Check sheet for the modelled part. Datum: model origin and axes. Units: mm. A direction names the side the tool comes from. Round coordinates to 2 decimals unless told otherwise and drop trailing zeros. Loops run counter-clockwise (first coordinate to the right, second up) from the corner with the lowest first, then second, coordinate; pieces in that order, holes last. Notation, with made-up numbers: (41, -25) - (93, -25) arc R30 ccw to (93, 13) - close; hole circle Ø11 at (75.5, 61). An arc over 180 degrees is marked (long way). Put each result on its own line as item: value.
```python
from build123d import *

# Parameters (mm, degrees)
F0_W     = 21.9964
F0_H     = 21.9964
F1_DEPTH = 101.6
F5_D     = 8.5
F5_DEPTH = 10
F5_TIP   = 2.5536576309
F7_D     = 8.5
F7_DEPTH = 10
F7_TIP   = 2.5536576309


with BuildPart() as f1:
    # F0 (on Front) → F1 (new body)
    with BuildSketch(Plane.XZ):
        Rectangle(F0_W, F0_H)
    extrude(amount=F1_DEPTH)

    # F2 (on Top) → F3 (revolve)
    with BuildSketch(Plane.XY):
        Polygon((-10.800095275, 0), (0, 0), (0, 24.9989666045), (-5.3329677321, 24.9989666045), (-10.800095275, 19.2432253866), (-10.800095275, 16.7330801487), (-12.0340296999, 16.7330801487), (-12.0340296999, 5.7621949818), (-10.800095275, 5.7621949818), align=None)
    revolve(axis=Axis((0, 12.4994833022, 0), (0, 1, 0)))

    # F5
    with Locations(Plane.YZ.offset(10.9982)):
        with Locations((-12.036957778, 0)):
            Hole(F5_D / 2, depth=F5_DEPTH)
            with Locations((0, 0, -(F5_DEPTH + F5_TIP / 2))):  # 118° drill point
                Cone(0, F5_D / 2, F5_TIP, mode=Mode.SUBTRACT)

    # F7
    with Locations(Plane.XZ.offset(101.6)):
        with Locations((0, 0)):
            Hole(F7_D / 2, depth=F7_DEPTH)
            with Locations((0, 0, -(F7_DEPTH + F7_TIP / 2))):  # 118° drill point
                Cone(0, F7_D / 2, F7_TIP, mode=Mode.SUBTRACT)


solid = f1.part
```
Item 1: Section check A-A on y = -71.5. Enter the section's corners in (x, z), then the cut area to 3 significant figures.
Filled sheet:
outline: (-11, -11) - (11, -11) - (11, 11) - (-11, 11) - close
area: 484 mm²
Item 2: Thickness scan on line 1 (X direction, y = -97.5, z = 0); line 2 (Y direction, x = -10.75, z = 3); line 3 (Z direction, x = 3, y = -57). Record the ranges inside material, lowest first. Write a range as from..to.
Filled sheet:
line 1: -11..-4.25, 4.25..11
line 2: -101.6..0, 5.76..16.73
line 3: -11..11
Item 3: Section check B-B on y = 1.5. Enter the section's corners in (x, z), then the cut area to 3 significant figures.
Filled sheet:
outline: circle Ø21.6 at (0, 0)
area: 366 mm²
Item 4: Go/stop test with flat-tipped pins: pin 1 (12 mm diameter, centred on x = 6.5, y = -4, fed in from +Z); pin 2 (4 mm diameter, centred on y = -85, z = 1.5, fed in from -X); pin 3 (1.5 mm diameter, centred on y = -32, z = -3, fed in from +X). Record where each tip stops, or that it passes through.
Filled sheet:
pin 1: z = 11
pin 2: x = -11
pin 3: x = 11
Item 5: Tool access check on faces 5 (the flat face through (-3.3, 0, -10.5)), 6 (the flat face through (-10.998, -50, 0)), 7 (the cylindrical face through (1.57, 11.17, 11.93)), 8 (the cylindrical face through (-2.285, -96.53, 3.584)). Record the directions out of +Z, -Z, +X, -X, +Y, -Y that give a thin tool (end or side, any length) a straight path to the whole face; none if there is none.
Filled sheet:
face 5: none
face 6: +Z, -Z, -X, -Y
face 7: +Y
face 8: -Y
Item 6: Release check for a two-part mould opening along Y. For faces 1 (the flat face through (0, -50, 10.998)), 2 (the flat face through (10, 5.762, 5)), 3 (the conical face through (-1.112, -12.623, -0.449)), 4 (the conical face through (1.23, 24.64, -5.54)) record: +Y half, -Y half, draft (parallel to the pull), parting line (faces both ways), or undercut.
Filled sheet:
face 1: draft
face 2: undercut
face 3: undercut
face 4: +Y half
